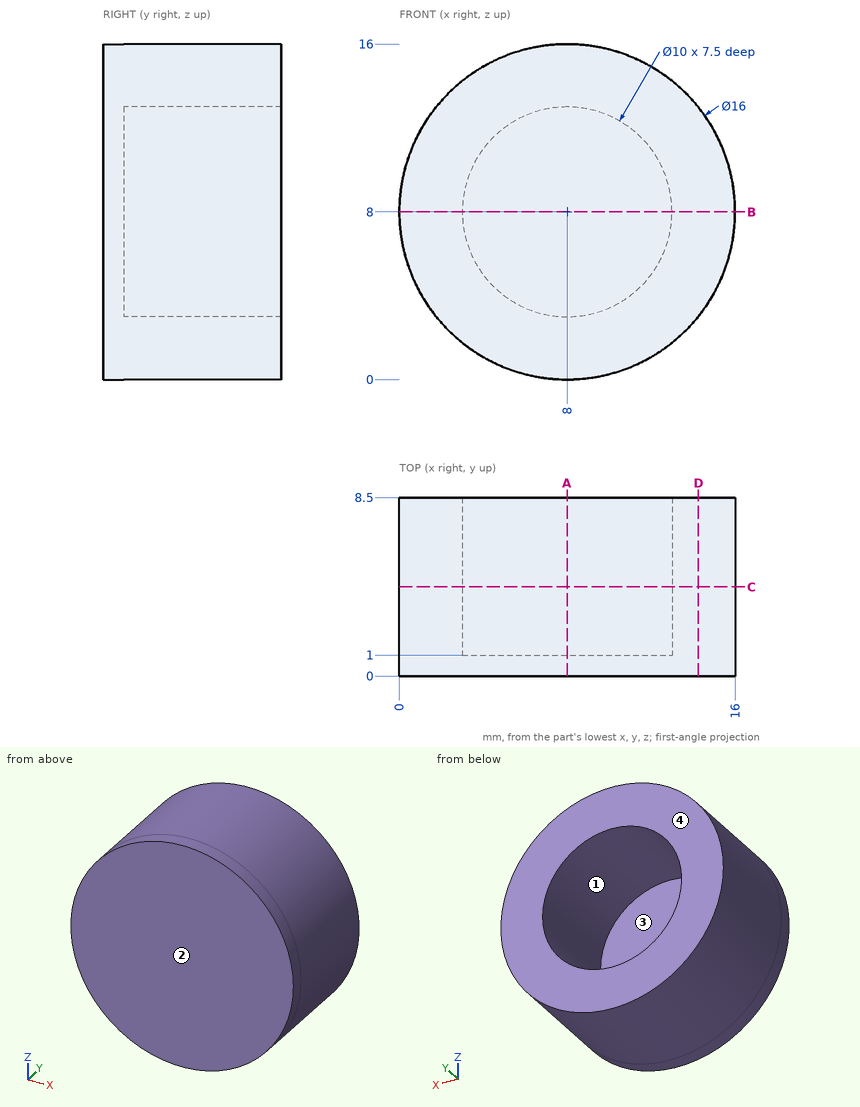
Print and shaded views of the part. All mm, measured from the part's lowest x, y and z. A direction names the side the tool comes from. Coordinates: 2 decimals unless noted, no trailing zeros. Write each loop counter-clockwise with the first axis right and the second up, starting at its lowest first coordinate (ties: lowest second). Pieces come first, ordered by that corner, then holes. Notation, with made-up numbers: (-13.75, 50) -> (-8.75, 50) arc R30 cw to (-8.75, 82) -> close; hole circle Ø3 at (-35, 17.25). An arc over 180 degrees is marked (long way). Use CSV: the item, a comma, the result in double quotes. Start each with the question number.
Q1. Cut at A-A, the plane x = 8. List the corners of the cut face in (y, z), then the cut area to 3 significant figures.
Q2. 3-axis set-ups, long thin cutter, end or side, ignore diameter. For the marked faces 1 and 2: which of +Z, -Z, +X, -X, +Y, -Y reach the whole face in a straight line?
Q3. Pull direction X, two halves, no side cores. Call the marked faces 3 and 4: released by +X, released by -X, zero draft, split by the parting line, or undercut.
Q4. Flat gauge pins, fed straight in: pin 1 Ø3 at (x, z) = (8, 9) entering from +Y; pin 2 Ø1 at (y, z) = (6.5, 2) entering from +X; pin 3 Ø4 at (y, z) = (4, 10.5) entering from +X. Where does each tip first touch, or does it go through?
Q5. Cut at B-B, the plane z = 8. List the corners of the cut face in (x, y).
Q6. Drill centre lines: probe 1 along Z at (x, y) = (8, 6.25); probe 2 along Y at (x, z) = (7.5, 3.75). Where is each one in solid material? Low to high.
Q7. Cut at D-D, the plane x = 14.25. List the corners of the cut face in (y, z), then the cut area to 3 significant figures.
Q8. Cut at C-C, the plane y = 4.25. List the corners of the cut face in (x, z).
Checked values:
1,outline,"(0, 0) -> (8.5, 0) -> (8.5, 3) -> (1, 3) -> (1, 13) -> (8.5, 13) -> (8.5, 16) -> (0, 16) -> close"
1,area,"61.0 mm²"
2,face 1,"+Y"
2,face 2,"+Z, -Z, +X, -X, -Y"
3,face 3,"undercut"
3,face 4,"zero draft"
4,pin 1,"stops at y = 1"
4,pin 2,"stops at x = 13.81"
4,pin 3,"stops at x = 15.98"
5,outline,"(0, 0) -> (16, 0) -> (16, 8.5) -> (13, 8.5) -> (13, 1) -> (3, 1) -> (3, 8.5) -> (0, 8.5) -> close"
6,probe 1,"z = 0 to 3, 13 to 16"
6,probe 2,"y = 0 to 1"
7,outline,"(0, 3.01) -> (8.5, 3.01) -> (8.5, 12.99) -> (0, 12.99) -> close"
7,area,"84.9 mm²"
8,outline,"circle Ø16 at (8, 8); hole circle Ø10 at (8, 8)"
